Design review of the part built by this model. Coordinates are the model's own, in mm. Face numbers are marked on the shaded views. A direction names the side the tool comes from. Round coordinates to 2 decimals unless told otherwise and drop trailing zeros. Loops run counter-clockwise (first coordinate to the right, second up) from the corner with the lowest first, then second, coordinate; pieces in that order, holes last. Notation, with made-up numbers: (72.5, 18) -> (113.5, 18) arc R37 cw to (113.5, 56) -> close; hole circle Ø3 at (65.25, -4). An arc over 180 degrees is marked (long way). Write each question's results on one line, items separated by ' | '. Start each with the question number.
from build123d import *

# Parameters (mm, degrees)
BOSS_EXTRU_1_DEPTH           = 176.25
ENL_V_MAT_EXTRU_1_DEPTH      = 374
ENL_V_MAT_EXTRU_2_REACH      = 440.777
BOSS_EXTRU_2_DEPTH           = 220
ENL_V_MAT_EXTRU_3_DEPTH      = 346.336158692
ENL_V_MAT_EXTRU_3_DEPTH_BACK = 346.336158692


with BuildPart() as part:
    # Esquisse1 → Boss.-Extru.1 (new, symmetric)
    with BuildSketch(Plane(origin=(0, 0, 0), x_dir=(1, 0, 0), z_dir=(0, 1, 0))):
        with BuildLine():
            Line((-205, 158), (205, 158))
            Line((205, 158), (205, -158))
            ThreePointArc((205, -158), (196, -162), (187, -158))
            Line((187, -158), (187, -151))
            Line((187, -151), (-187, -151))
            Line((-187, -151), (-187, -158))
            ThreePointArc((-187, -158), (-196, -162), (-205, -158))
            Line((-205, -158), (-205, 158))
        make_face()
    extrude(amount=BOSS_EXTRU_1_DEPTH, both=True)

    # Esquisse2 → Enlèv. mat.-Extru.1 (cut)
    with BuildSketch(Plane(origin=(-187, 0, 0), x_dir=(0, 0, -1), z_dir=(1, 0, 0))):
        with BuildLine():
            Line((-151, -97.25), (-151, -176.25))
            Line((-151, -176.25), (-128, -176.25))
            Line((-128, -176.25), (-128, -106.25))
            Line((-128, -106.25), (-147, -106.25))
            ThreePointArc((-147, -106.25), (-149.954965027, -102.174428901), (-151, -97.25))
        make_face()
        with BuildLine():
            Line((-151, 40.75), (-151, -97.25))
            ThreePointArc((-151, -97.25), (-149.954965027, -92.325571099), (-147, -88.25))
            Line((-147, -88.25), (140, -88.25))
            Line((140, -88.25), (140, 36.75))
            Line((140, 36.75), (-149, 36.75))
            ThreePointArc((-149, 36.75), (-150.472135955, 38.513932023), (-151, 40.75))
        make_face()
        with BuildLine():
            Line((-148, 176.25), (-151, 176.25))
            Line((-151, 176.25), (-151, 169.25))
            ThreePointArc((-151, 169.25), (-150.218401957, 173.057886553), (-148, 176.25))
        make_face()
    extrude(amount=ENL_V_MAT_EXTRU_1_DEPTH, mode=Mode.SUBTRACT)

    # Enlèv. mat.-Extru.2: up to this face of the body (flat: up to its plane)
    enl_v_mat_extru_2_end = Plane(part.part.faces().sort_by_distance((0, 36.75, 4.5))[0])
    # Esquisse3 → Enlèv. mat.-Extru.2 (cut, up to the picked face)
    with BuildSketch(Plane(origin=(0, 176.25, 0), x_dir=(1, 0, 0), z_dir=(0, 1, 0)), mode=Mode.PRIVATE) as enl_v_mat_extru_2_sk1:
        with BuildLine():
            Line((-187, -151), (-187, -142))
            ThreePointArc((-187, -142), (-186.230249471, -146.74341649), (-184, -151))
            Line((-184, -151), (-187, -151))
        make_face()
    enl_v_mat_extru_2_tool1 = split(extrude(enl_v_mat_extru_2_sk1.sketch, amount=-ENL_V_MAT_EXTRU_2_REACH, mode=Mode.PRIVATE), bisect_by=enl_v_mat_extru_2_end, keep=Keep.BOTH, mode=Mode.PRIVATE)
    # Esquisse3 → Enlèv. mat.-Extru.2 (cut, up to the picked face)
    with BuildSketch(Plane(origin=(0, 176.25, 0), x_dir=(1, 0, 0), z_dir=(0, 1, 0)), mode=Mode.PRIVATE) as enl_v_mat_extru_2_sk2:
        with BuildLine():
            Line((184, -151), (187, -151))
            Line((187, -151), (187, -142))
            ThreePointArc((187, -142), (186.230249471, -146.74341649), (184, -151))
        make_face()
    enl_v_mat_extru_2_tool2 = split(extrude(enl_v_mat_extru_2_sk2.sketch, amount=-ENL_V_MAT_EXTRU_2_REACH, mode=Mode.PRIVATE), bisect_by=enl_v_mat_extru_2_end, keep=Keep.BOTH, mode=Mode.PRIVATE)
    add(enl_v_mat_extru_2_tool1.solids().sort_by(Axis((-186.117852, 176.25, 148.797484), (0, -1, 0)))[0], mode=Mode.SUBTRACT)
    add(enl_v_mat_extru_2_tool2.solids().sort_by(Axis((186.117852, 176.25, 148.797484), (0, -1, 0)))[0], mode=Mode.SUBTRACT)

    # Esquisse4 → Boss.-Extru.2 (add, symmetric)
    with BuildSketch(Plane(origin=(0, 0, 0), x_dir=(0, 0, -1), z_dir=(1, 0, 0))):
        with BuildLine():
            Line((158, 176.25), (-178, 176.25))
            ThreePointArc((-178, 176.25), (-182, 185.25), (-178, 194.25))
            Line((-178, 194.25), (158, 194.25))
            Line((158, 194.25), (158, 176.25))
        make_face()
    extrude(amount=BOSS_EXTRU_2_DEPTH, both=True)

    # Esquisse5 → Enlèv. mat.-Extru.3 (cut, two sides: drawn at the far end of the back side and taken through both)
    with BuildSketch(Plane.XY.offset(-ENL_V_MAT_EXTRU_3_DEPTH_BACK)):
        with BuildLine():
            Line((220, 194.25), (216, 194.25))
            ThreePointArc((216, 194.25), (218.954965027, 190.174428901), (220, 185.25))
            Line((220, 185.25), (220, 194.25))
        make_face()
        with BuildLine():
            ThreePointArc((-220, 185.25), (-218.954965027, 190.174428901), (-216, 194.25))
            Line((-216, 194.25), (-220, 194.25))
            Line((-220, 194.25), (-220, 185.25))
        make_face()
        with BuildLine():
            ThreePointArc((-216, 176.25), (-218.954965027, 180.325571099), (-220, 185.25))
            Line((-220, 185.25), (-220, 176.25))
            Line((-220, 176.25), (-216, 176.25))
        make_face()
        with BuildLine():
            Line((220, 176.25), (220, 185.25))
            ThreePointArc((220, 185.25), (218.954965027, 180.325571099), (216, 176.25))
            Line((216, 176.25), (220, 176.25))
        make_face()
    extrude(amount=ENL_V_MAT_EXTRU_3_DEPTH + ENL_V_MAT_EXTRU_3_DEPTH_BACK, mode=Mode.SUBTRACT)

    # Esquisse6 → Révolution1 (revolve)
    with BuildSketch(Plane(origin=(0, 0, 0), x_dir=(0, 0, -1), z_dir=(1, 0, 0)), mode=Mode.PRIVATE) as r_volution1_sk:
        with BuildLine():
            Line((-151, 111.25), (-162, 111.25))
            ThreePointArc((-162, 111.25), (-166.242640687, 113.007359313), (-168, 117.25))
            Line((-168, 117.25), (-168, 118.25))
            ThreePointArc((-168, 118.25), (-172.862133877, 117.576087333), (-177.588231263, 116.25))
            ThreePointArc((-177.588231263, 116.25), (-178.611504042, 115.474039518), (-179, 114.25))
            Line((-179, 114.25), (-179, 101.25))
            Line((-179, 101.25), (-151, 101.25))
            Line((-151, 101.25), (-151, 111.25))
        make_face()
    revolve(r_volution1_sk.sketch.rotate(Axis((0, 101.25, 201.29718837), (0, 0, -1)), 90), axis=Axis((0, 101.25, 201.29718837), (0, 0, -1)))


solid = part.part
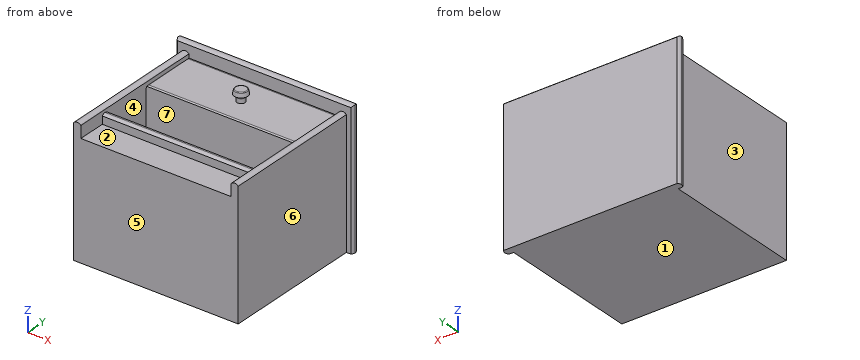
1) To check wall thickness, follow line 1 (Y direction, x = -176.5, z = -106); line 2 (X direction, y = -14, z = -64.5); line 3 (Y direction, x = 36.5, z = 137). State the ranges of each line that lie inside material, in increasing order. Write a range as from..to.
2) The part is to be moulded in two halves that separate along Y. For the marked faces 4, 5, 6 and 7, say which applies: +Y half, -Y half, draft (parallel to the pull), parting line (faces both ways), or undercut.
3) Take a section at B-B (y = -67). Write out the cut boundary in (x, z) (3 decimals).
4) Insertion check: pin 1 (9.5 mm diameter, centred on x = -12.5, z = 137, fed in from -Y); pin 2 (5 mm diameter, centred on y = 134.5, z = -68, fed in from -X); pin 3 (8 mm diameter, centred on x = -3, y = 107, fed in from +Z). Each pin has a flat end and moves straight along its axis. Give the tip position at first contact, or say it passes through.
5) Take a section at A-A (z = -58). Write out the cut boundary in (x, y) (3 decimals), plus the area to 3 significant figures.
6) For the marked faces 1, 2 and 3, list the 3-axis set-ups (+Z, -Z, +X, -X, +Y, -Y) from which the entire face can be reached by the end or side of a thin tool; tool diameter is ignored.
7) Take a section at C-C (x = -135). Write out the cut boundary in (y, z) (3 decimals), plus the area to 3 significant figures.
8) Take a section at D-D (y = 70.5). Write out the cut boundary in (x, z) (3 decimals), plus the area to 3 significant figures.
Geometry check:
1) line 1: y = -176.25..-88.25, 36.75..194.25 | line 2: x = -205..-187, 187..205 | line 3: y = -106.25..-88.25, 36.75..194.25
2) face 4: undercut | face 5: -Y half | face 6: draft | face 7: undercut
3) outline: (-205, -158) -> (205, -158) -> (205, 158) arc R12.125 ccw to (187, 158) -> (187, -140) -> (-187, -140) -> (-187, 158) arc R12.125 ccw to (-205, 158) -> close
4) pin 1: stops at y = -106.25 | pin 2: stops at x = -205 | pin 3: stops at z = 179
5) outline: (-216, 176.25) -> (-205, 176.25) -> (-205, -176.25) -> (205, -176.25) -> (205, 176.25) -> (216, 176.25) arc R12.125 ccw to (216, 194.25) -> (-216, 194.25) arc R12.125 ccw to start; hole (-187, -88.25) -> (187, -88.25) -> (187, 36.75) -> (-187, 36.75) -> close | area: 106,000 mm^2
6) face 1: -Z, +X, -X, +Y, -Y | face 2: +Z, -Y | face 3: +Z, -Z, -X, -Y
7) outline: (-176.25, -158) -> (194.25, -158) -> (194.25, 178) arc R12.125 ccw to (176.25, 178) -> (176.25, 148) arc R9.667 ccw to (169.25, 151) -> (40.75, 151) arc R5 ccw to (36.75, 149) -> (36.75, -140) -> (-88.25, -140) -> (-88.25, 147) arc R12.125 ccw to (-106.25, 147) -> (-106.25, 128) -> (-176.25, 128) -> close | area: 77,000 mm^2
8) outline: (-205, -158) -> (205, -158) -> (205, 158) arc R12.125 ccw to (187, 158) -> (187, 142) arc R15 ccw to (184, 151) -> (-184, 151) arc R15 ccw to (-187, 142) -> (-187, 158) arc R12.125 ccw to (-205, 158) -> close | area: 127,000 mm^2
